For this review, use the dimensioned drawing (mm, ordinates from the lowest corner) and the shaded views. Round coordinates to 2 decimals unless told otherwise and drop trailing zeros. Order: outer loops, then holes, each group sorted by start corner. A loop starts at its lowest first (then second) coordinate and runs counter-clockwise, first axis right, second up. Notation, with made-up numbers: (-34, -22) - (-21, -22) arc R7 ccw to (-21, -9) - close; hole circle Ø1 at (70.25, -2). An arc over 180 degrees is marked (long way). Write each question's results on one line, items separated by ' | '. Start each with the question number.
(1) Take a section at D-D, the plane z = 75.5. Give the boundary of the cut face in (x, y) (1 decimal), plus the area to 3 significant figures.
(2) Take a section at A-A, the plane x = 39.5. Give the boundary of the cut face in (y, z) (3 decimals), plus the area to 3 significant figures.
(3) Take a section at C-C, the plane y = 2.25. Give the boundary of the cut face in (x, z) (3 decimals), plus the area to 3 significant figures.
(4) Insertion check: pin 1 Ø4.5 at (x, z) = (83.39, 16.94) entering from -Y; pin 2 Ø1.5 at (x, y) = (28, 2) entering from -Z; pin 3 Ø1.5 at (x, y) = (41.5, 2) entering from -Z; pin 4 Ø2.5 at (x, z) = (16.94, 83.39) entering from -Y. Each pin has a flat end and moves straight along its axis. Give the tip position at first contact, or say it passes through.
(5) For L1, parallel to X at y = 2.05, z = 83.5; L2, parallel to Z at x = 17, y = 2.9; L3, parallel to X at y = 0.5, z = 17.5, list the stretches that pass through material, from the lowest coordinate up. Write a range as from..to.
(6) Take a section at B-B, the plane z = 38. Give the boundary of the cut face in (x, y) (3 decimals).
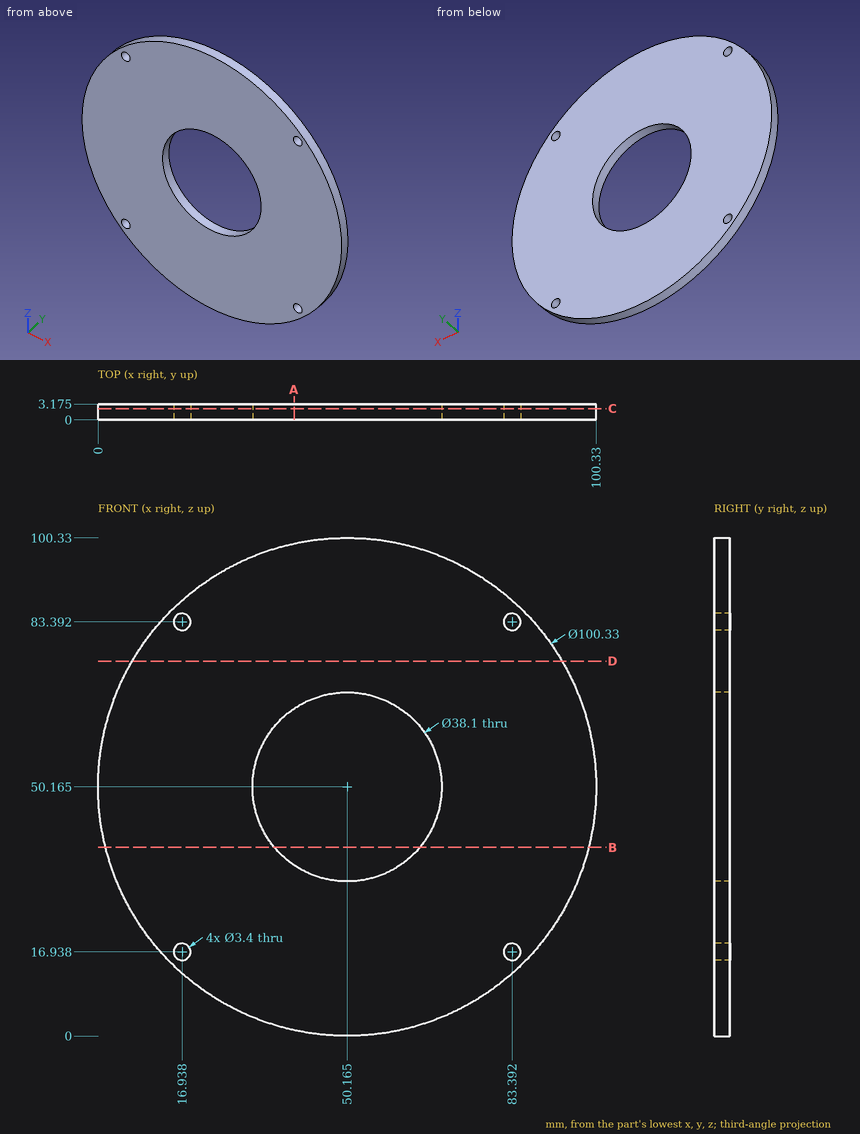
Results below:
1) outline: (6.9, 0) - (93.5, 0) - (93.5, 3.2) - (6.9, 3.2) - close | area: 275 mm^2
2) outline: (0, 1.147) - (3.175, 1.147) - (3.175, 34.38) - (0, 34.38) - close; (0, 65.95) - (3.175, 65.95) - (3.175, 99.183) - (0, 99.183) - close | area: 211 mm^2
3) outline: circle Ø100.33 at (50.165, 50.165); hole circle Ø3.4 at (16.938, 16.938); hole circle Ø3.4 at (16.938, 83.392); hole circle Ø38.1 at (50.165, 50.165); hole circle Ø3.4 at (83.392, 16.938); hole circle Ø3.4 at (83.392, 83.392) | area: 6,730 mm^2
4) pin 1: stops at y = 0 | pin 2: stops at z = 4.8 | pin 3: stops at z = 0.63 | pin 4: passes through
5) L1: x = 12.68..15.24, 18.63..81.7, 85.09..87.65 | L2: z = 12.53..15.24, 18.64..81.69, 85.09..87.8 | L3: x = 12.09..15.33, 18.54..81.79, 85..88.24
6) outline: (1.497, 0) - (35.505, 0) - (35.505, 3.175) - (1.497, 3.175) - close; (64.825, 0) - (98.833, 0) - (98.833, 3.175) - (64.825, 3.175) - close
